The model under review builds one solid part; all positions refer to its coordinate system, in mm. Coordinates: 2 decimals unless noted, no trailing zeros. Write each loop counter-clockwise with the first axis right and the second up, starting at its lowest first coordinate (ties: lowest second). Pieces come first, ordered by that corner, then holes. Notation, with made-up numbers: (-2.75, 43) - (15.25, 43) arc R12 ccw to (15.25, 49) - close; hole circle Ø3 at (20.5, -5). An arc over 180 degrees is marked (long way). Return JSON: item names as keys, results as strings. Group by question number.
(1) We need section B-B on y = -4. State the section outline as (x, z) points.
(2) We need section C-C on z = 320. State the section outline as (x, y) points, then the cut area to 3 significant figures.
(3) To check wall thickness, follow L1, parallel to X at y = -14.6, z = 20; L2, parallel to Y at x = 8, z = 456; L3, parallel to Z at x = 0, y = 14.45. State the ranges of each line that lie inside material, in increasing order. Write a range as from..to.
(4) We need section D-D on x = 0. Give the number of separate pieces and of enclosed holes in the cut face, then the cut area to 3 significant figures.
(5) We need section A-A on z = 61. State the section outline as (x, y) points.
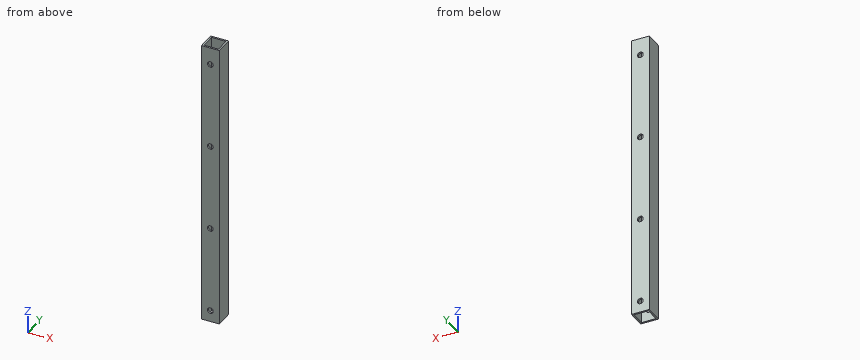
```python
from build123d import *

# Parameters (mm, degrees)
F0_W          = 31
F0_H          = 31
F0_W_2        = 25
F0_H_2        = 25
F1_DEPTH      = 500
F2_R          = 5
F3_DEPTH      = 15.501
F3_DEPTH_BACK = 15.501


with BuildPart() as f1:
    # F0 (on Top) → F1 (new body)
    with BuildSketch(Plane.XY):
        Rectangle(F0_W, F0_H)
        Rectangle(F0_W_2, F0_H_2, mode=Mode.SUBTRACT)
    extrude(amount=F1_DEPTH)

    # F2 (on Front) → F3 (cut, two sides)
    with BuildSketch(Plane.XZ) as f3_sk:
        with Locations((0, 470)):
            Circle(F2_R)
        with Locations((0, 320)):
            Circle(F2_R)
        with Locations((0, 170)):
            Circle(F2_R)
        with Locations((0, 20)):
            Circle(F2_R)
    extrude(amount=F3_DEPTH, mode=Mode.SUBTRACT)
    extrude(f3_sk.sketch, amount=-F3_DEPTH_BACK, mode=Mode.SUBTRACT)


solid = f1.part
```
Ans:
{
 "1": {"outline": "(-15.5, 0) - (-12.5, 0) - (-12.5, 500) - (-15.5, 500) - close; (12.5, 0) - (15.5, 0) - (15.5, 500) - (12.5, 500) - close"},
 "2": {"outline": "(-15.5, -15.5) - (-5, -15.5) - (-5, -12.5) - (-12.5, -12.5) - (-12.5, 12.5) - (-5, 12.5) - (-5, 15.5) - (-15.5, 15.5) - close; (5, -15.5) - (15.5, -15.5) - (15.5, 15.5) - (5, 15.5) - (5, 12.5) - (12.5, 12.5) - (12.5, -12.5) - (5, -12.5) - close", "area": "276 mm²"},
 "3": {"L1": "-15.5..-5, 5..15.5", "L2": "-15.5..-12.5, 12.5..15.5", "L3": "0..15, 25..165, 175..315, 325..465, 475..500"},
 "4": {"separate pieces": "10", "enclosed holes": "0", "area": "2,760 mm²"},
 "5": {"outline": "(-15.5, -15.5) - (15.5, -15.5) - (15.5, 15.5) - (-15.5, 15.5) - close; hole (-12.5, -12.5) - (12.5, -12.5) - (12.5, 12.5) - (-12.5, 12.5) - close"}
}
